Source: CAD feature listing. Evaluate the final solid. Frame: model axes, mm. A direction names the side the tool comes from. Give positions to 0.01 mm unless a question says otherwise; leave off trailing zeros. Write each loop counter-clockwise with the first axis right and the second up, starting at its lowest first coordinate (ties: lowest second). Pieces come first, ordered by that corner, then holes. Notation, with made-up numbers: (10, -7.5) -> (14, -7.5) arc R18 ccw to (14, 3.5) -> close; hole circle Ø2 at (84.25, 60). An arc over 180 degrees is marked (long way). Write item = value, one per line.
from build123d import *

# Parameters (mm, degrees)
SKETCH1_W                    = 75
SKETCH1_H                    = 139.2
SKETCH1_R                    = 1.1
SKETCH1_W_2                  = 55
SKETCH1_H_2                  = 119.2
BOSS_EXTRUDE1_DEPTH          = 0.8
BOSS_EXTRUDE1_DEPTH_BACK     = 0.8
SKETCH2_W                    = 20
SKETCH2_H                    = 10
BOSS_EXTRUDE2_DEPTH          = 1.6
SKETCH6_W                    = 125
SKETCH6_H                    = 75.4
SKETCH6_W_2                  = 105
SKETCH6_H_2                  = 55.4
BOSS_EXTRUDE4_DEPTH          = 1.6
M2_5_CLEARANCE_HOLE1_D       = 2.9
M2_5_CLEARANCE_HOLE1_DEPTH   = 11.5
FILLET1_R                    = 1.5
CUT_EXTRUDE2_DEPTH           = 10
SKETCH10_W                   = 55
SKETCH10_H                   = 10
BOSS_EXTRUDE5_DEPTH          = 1.6
SKETCH11_W                   = 19
SKETCH11_H                   = 8
SKETCH11_R                   = 1.45
BOSS_EXTRUDE6_DEPTH          = 1.6
SKETCH12_W                   = 55
SKETCH12_H                   = 8
BOSS_EXTRUDE7_DEPTH          = 1.6
FILLET3_R                    = 2
CHAMFER1_SIZE                = 5
SKETCH13_R                   = 1.5
CUT_EXTRUDE3_DEPTH           = 10
SKETCH15_R                   = 1.55
CUT_EXTRUDE4_DEPTH           = 10
CHAMFER2_SIZE                = 5
FILLET4_R                    = 2
SKETCH17_W                   = 58.67264252
SKETCH17_H                   = 24.596391624
SKETCH17_W_2                 = 62.115544984
SKETCH17_H_2                 = 8.350438831
BOSS_EXTRUDE8_DEPTH          = 1.6
SKETCH18_R                   = 0.85
CUT_EXTRUDE5_DEPTH           = 10
M2_CLEARANCE_HOLE1_D         = 2.4
M2_CLEARANCE_HOLE1_DEPTH     = 10
ESQUISSE1_R                  = 0.9
ENL_V_MAT_EXTRU_1_DEPTH      = 10
ENL_V_MAT_EXTRU_1_DEPTH_BACK = 10


with BuildPart() as part:
    # Sketch1 → Boss-Extrude1 (new body, two sides)
    with BuildSketch(Plane(origin=(0, 0, 0), x_dir=(1, 0, 0), z_dir=(0, 1, 0))) as boss_extrude1_sk:
        Rectangle(SKETCH1_W, SKETCH1_H)
        with Locations((-26.35, 64.6)):
            Circle(SKETCH1_R, mode=Mode.SUBTRACT)
        with Locations((26.35, 64.6)):
            Circle(SKETCH1_R, mode=Mode.SUBTRACT)
        with Locations((26.35, -64.6)):
            Circle(SKETCH1_R, mode=Mode.SUBTRACT)
        with Locations((-26.35, -64.6)):
            Circle(SKETCH1_R, mode=Mode.SUBTRACT)
        Rectangle(SKETCH1_W_2, SKETCH1_H_2, mode=Mode.SUBTRACT)
    extrude(amount=BOSS_EXTRUDE1_DEPTH)
    extrude(boss_extrude1_sk.sketch, amount=-BOSS_EXTRUDE1_DEPTH_BACK)

    # Sketch2 → Boss-Extrude2 (add)
    with BuildSketch(Plane(origin=(0, 0.8, 0), x_dir=(1, 0, 0), z_dir=(0, 1, 0))):
        with Locations((47.5, 49.6)):
            Rectangle(SKETCH2_W, SKETCH2_H)
        with Locations((-47.5, 49.6)):
            Rectangle(SKETCH2_W, SKETCH2_H)
        with Locations((47.5, -20.4)):
            Rectangle(SKETCH2_W, SKETCH2_H)
        with Locations((-47.5, -20.4)):
            Rectangle(SKETCH2_W, SKETCH2_H)
    extrude(amount=-BOSS_EXTRUDE2_DEPTH)

    # Sketch6 → Boss-Extrude4 (add)
    with BuildSketch(Plane(origin=(0, 0.8, 0), x_dir=(1, 0, 0), z_dir=(0, 1, 0))):
        with Locations((0, 82.3)):
            Rectangle(SKETCH6_W, SKETCH6_H)
        with Locations((0, 82.3)):
            Rectangle(SKETCH6_W_2, SKETCH6_H_2, mode=Mode.SUBTRACT)
    extrude(amount=-BOSS_EXTRUDE4_DEPTH)

    # M2.5 Clearance Hole1
    with Locations(Plane(origin=(0, 0.8, 0), x_dir=(-1, 0, 0), z_dir=(0, 1, 0))):
        with Locations((-52.5, -49.6), (-52.5, 20.4), (-42.5, -49.6), (-42.5, 20.4)):
            m2_5_clearance_hole1 = Hole(M2_5_CLEARANCE_HOLE1_D / 2, depth=M2_5_CLEARANCE_HOLE1_DEPTH)

    # Mirror1: M2.5 Clearance Hole1 across plane
    add(m2_5_clearance_hole1.mirror(Plane(origin=(0, 0, 0), x_dir=(0, 0, 1), z_dir=(1, 0, 0))), mode=Mode.SUBTRACT)

    # Fillet1
    fillet1_edges = [part.edges().sort_by_distance(p)[0] for p in [
        (37.5, 0, 25.4),
        (37.5, 0, 15.4),
        (-37.5, 0, 15.4),
        (-37.5, 0, 25.4),
        (-37.5, 0, -44.6),
        (37.5, 0, -44.6),
        (27.5, 0, -59.6),
        (-27.5, 0, -59.6),
        (27.5, 0, -54.6),
        (-27.5, 0, -54.6),
    ]]
    fillet(fillet1_edges, radius=FILLET1_R)

    # Sketch9 → Cut-Extrude2 (cut)
    with BuildSketch(Plane(origin=(0, 0.8, 0), x_dir=(1, 0, 0), z_dir=(0, 1, 0))):
        with BuildLine():
            Line((-25.25, -63.1), (-25.25, -66.1))
            ThreePointArc((-25.25, -66.1), (-26.35, -67.2), (-27.45, -66.1))
            Line((-27.45, -66.1), (-27.45, -63.1))
            ThreePointArc((-27.45, -63.1), (-26.35, -62), (-25.25, -63.1))
        make_face()
    cut_extrude2 = extrude(amount=-CUT_EXTRUDE2_DEPTH, mode=Mode.SUBTRACT)

    # Mirror2: Cut-Extrude2 across plane
    add(cut_extrude2.mirror(Plane(origin=(0, 0, 0), x_dir=(0, 0, 1), z_dir=(1, 0, 0))), mode=Mode.SUBTRACT)

    # Sketch10 → Boss-Extrude5 (add)
    with BuildSketch(Plane(origin=(0, 0.8, 0), x_dir=(1, 0, 0), z_dir=(0, 1, 0))):
        with Locations((0, -20.4)):
            Rectangle(SKETCH10_W, SKETCH10_H)
    extrude(amount=-BOSS_EXTRUDE5_DEPTH)

    # Sketch11 → Boss-Extrude6 (add)
    with BuildSketch(Plane(origin=(0, 0.8, 0), x_dir=(1, 0, 0), z_dir=(0, 1, 0))):
        with Locations((-37, 5.6)):
            Rectangle(SKETCH11_W, SKETCH11_H)
        with Locations((37, 5.6)):
            Rectangle(SKETCH11_W, SKETCH11_H)
        with Locations((42.5, 5.6)):
            Circle(SKETCH11_R, mode=Mode.SUBTRACT)
    extrude(amount=-BOSS_EXTRUDE6_DEPTH)

    # Sketch12 → Boss-Extrude7 (add)
    with BuildSketch(Plane(origin=(0, 0.8, 0), x_dir=(1, 0, 0), z_dir=(0, 1, 0))):
        with Locations((0, 5.6)):
            Rectangle(SKETCH12_W, SKETCH12_H)
    extrude(amount=-BOSS_EXTRUDE7_DEPTH)

    # Fillet3
    fillet3_edges = [part.edges().sort_by_distance(p)[0] for p in [
        (37.5, 0, -1.6),
        (-37.5, 0, -1.6),
    ]]
    fillet(fillet3_edges, radius=FILLET3_R)

    # Chamfer1
    chamfer1_edges = [part.edges().sort_by_distance(p)[0] for p in [
        (62.5, 0, -44.6),
        (62.5, 0, -120),
        (-62.5, 0, -120),
        (-62.5, 0, -44.6),
    ]]
    chamfer(chamfer1_edges, length=CHAMFER1_SIZE)

    # Sketch13 → Cut-Extrude3 (cut)
    with BuildSketch(Plane(origin=(0, 0.8, 0), x_dir=(1, 0, 0), z_dir=(0, 1, 0))):
        with Locations((-51.439339828, 108.939339828)):
            Circle(SKETCH13_R)
        with Locations((51.439339828, 108.939339828)):
            Circle(SKETCH13_R)
    extrude(amount=-CUT_EXTRUDE3_DEPTH, mode=Mode.SUBTRACT)

    # Sketch15 → Cut-Extrude4 (cut)
    with BuildSketch(Plane.XZ.offset(0.8)):
        with Locations((37, -5.6)):
            Circle(SKETCH15_R)
    cut_extrude4 = extrude(amount=-CUT_EXTRUDE4_DEPTH, mode=Mode.SUBTRACT)

    # Mirror3: Cut-Extrude4 across plane
    add(cut_extrude4.mirror(Plane(origin=(0, 0, 0), x_dir=(0, 0, 1), z_dir=(1, 0, 0))), mode=Mode.SUBTRACT)

    # Chamfer2
    chamfer2_edges = [part.edges().sort_by_distance(p)[0] for p in [
        (-27.5, 0, 59.6),
        (27.5, 0, 59.6),
        (52.5, 0, -54.6),
        (37.5, 0, -54.6),
        (-37.5, 0, -54.6),
        (-52.5, 0, -54.6),
        (27.5, 0, -44.6),
        (-27.5, 0, -44.6),
        (-27.5, 0, 15.4),
        (27.5, 0, 15.4),
        (27.5, 0, 25.4),
        (-27.5, 0, 25.4),
        (-27.5, 0, -9.6),
        (27.5, 0, -9.6),
        (27.5, 0, -1.6),
        (-27.5, 0, -1.6),
    ]]
    chamfer(chamfer2_edges, length=CHAMFER2_SIZE)

    # Fillet4
    fillet4_edges = [part.edges().sort_by_distance(p)[0] for p in [
        (-27.5, 0, 30.4),
        (-22.5, 0, 25.4),
        (-22.5, 0, -1.6),
        (-27.5, 0, 3.4),
        (-22.5, 0, 15.4),
        (-27.5, 0, 10.4),
        (-22.5, 0, -9.6),
        (-27.5, 0, -14.6),
        (-27.5, 0, -39.6),
        (-22.5, 0, -44.6),
        (37.5, 0, -59.6),
        (42.5, 0, -54.6),
        (47.5, 0, -54.6),
        (52.5, 0, -59.6),
        (22.5, 0, -44.6),
        (27.5, 0, -39.6),
        (22.5, 0, -9.6),
        (27.5, 0, -14.6),
        (22.5, 0, 15.4),
        (27.5, 0, 10.4),
        (27.5, 0, 3.4),
        (22.5, 0, -1.6),
        (27.5, 0, 30.4),
        (22.5, 0, 25.4),
        (22.5, 0, 59.6),
        (27.5, 0, 54.6),
        (-27.5, 0, 54.6),
        (-22.5, 0, 59.6),
        (-52.5, 0, -59.6),
        (-47.5, 0, -54.6),
        (-42.5, 0, -54.6),
        (-37.5, 0, -59.6),
    ]]
    fillet(fillet4_edges, radius=FILLET4_R)

    # Sketch17 → Boss-Extrude8 (add)
    with BuildSketch(Plane(origin=(0, 0.8, 0), x_dir=(1, 0, 0), z_dir=(0, 1, 0))):
        with Locations((0.384318619, -6.570339181)):
            Rectangle(SKETCH17_W, SKETCH17_H)
        with Locations((0.147528901, 56.270374441)):
            Rectangle(SKETCH17_W_2, SKETCH17_H_2)
    extrude(amount=-BOSS_EXTRUDE8_DEPTH)

    # Sketch18 → Cut-Extrude5 (cut)
    with BuildSketch(Plane(origin=(0, 0.8, 0), x_dir=(1, 0, 0), z_dir=(0, 1, 0))):
        with Locations((-37.5, 10.45)):
            Circle(SKETCH18_R)
        with Locations((37.5, 10.45)):
            Circle(SKETCH18_R)
    extrude(amount=-CUT_EXTRUDE5_DEPTH, mode=Mode.SUBTRACT)

    # M2 Clearance Hole1
    with Locations(Plane.XZ.offset(0.8)):
        with Locations((33.75, -65.6), (-33.75, -65.6)):
            Hole(M2_CLEARANCE_HOLE1_D / 2, depth=M2_CLEARANCE_HOLE1_DEPTH)

    # Esquisse1 → Enl_v. mat.-Extru.1 (cut, two sides)
    with BuildSketch(Plane.XZ.offset(0.8)) as enl_v_mat_extru_1_sk:
        with Locations((42.5, -115)):
            Circle(ESQUISSE1_R)
        with Locations((-42.5, -115)):
            Circle(ESQUISSE1_R)
    extrude(amount=ENL_V_MAT_EXTRU_1_DEPTH, mode=Mode.SUBTRACT)
    extrude(enl_v_mat_extru_1_sk.sketch, amount=-ENL_V_MAT_EXTRU_1_DEPTH_BACK, mode=Mode.SUBTRACT)


solid = part.part
(1) Section query B-B (z = -87). Return loops of the section in (x, y), plus the area to 3 significant figures.
Values follow:
outline = (-62.5, -0.8) -> (-52.5, -0.8) -> (-52.5, 0.8) -> (-62.5, 0.8) -> close; (52.5, -0.8) -> (62.5, -0.8) -> (62.5, 0.8) -> (52.5, 0.8) -> close
area = 32.0 mm2
(2) Section query D-D (y = 0.15). Give the number of separate pieces and of enclosed holes in the cut face, plus the area to 3 significant figures.
Values follow:
separate_pieces = 1
enclosed_holes = 22
area = 10,000 mm2
(3) Material intervals for line 1 (Z direction, x = -2, y = 0.65); line 2 (X direction, y = 0.4, z = 37); line 3 (X direction, y = 0.1, z = -115), sorted ascending.
Values follow:
line_1 = -120 to -110, -69.6 to -44.6, -9.6 to 25.4, 59.6 to 69.6
line_2 = -37.5 to -27.5, 27.5 to 37.5
line_3 = -62.5 to -43.4, -41.6 to 41.6, 43.4 to 62.5
(4) First-contact query: pin 1 (1.4 mm diameter, centred on x = 33.75, z = -65.6, fed in from -Y); pin 2 (0.5 mm diameter, centred on y = 0, z = -24, fed in from -X); pin 3 (0.8 mm diameter, centred on y = 0, z = 40.5, fed in from +X); pin 4 (0.8 mm diameter, centred on x = 46, y = 0, fed in from +Z). Flat tips, straight axial feed; report the tip coordinate or a pass-through.
Values follow:
pin_1 = through
pin_2 = -37.5
pin_3 = 37.5
pin_4 = 25.4
(5) Pull-direction query (Z, two-part tool) for faces 3 (the face through (-60, 0, -117.5)), 4 (the face through (-1, -0.8, -48)), 5 (the face through (25, 0, 57.1)); classes: pulls with the +Z half, pulls with the -Z half, needs draft (parallel to the pull), parting line crosses it, or undercut.
Values follow:
face_3 = pulls with the -Z half
face_4 = needs draft
face_5 = undercut
(6) Section query C-C (x = 8). Return loops of the section in (y, z).
Values follow:
outline = (-0.8, -120) -> (0.8, -120) -> (0.8, -110) -> (-0.8, -110) -> close; (-0.8, -69.6) -> (0.8, -69.6) -> (0.8, -44.6) -> (-0.8, -44.6) -> close; (-0.8, -9.6) -> (0.8, -9.6) -> (0.8, 25.4) -> (-0.8, 25.4) -> close; (-0.8, 59.6) -> (0.8, 59.6) -> (0.8, 69.6) -> (-0.8, 69.6) -> close
(7) Access query for faces 1 (the face through (60, 0, -117.5)), 2 (the face through (40, 0, -57.1)). Directions: +Z, -Z, +X, -X, +Y, -Y. A direction counts if a zero-diameter tool reaches every point of the face in a straight line with its end or side. Return the directions, or none.
Values follow:
face_1 = -Z, +X, +Y, -Y
face_2 = +Y, -Y
(8) Section query A-A (x = -29.5). Return loops of the section in (y, z).
Values follow:
outline = (-0.8, -120) -> (0.8, -120) -> (0.8, -110) -> (-0.8, -110) -> close; (-0.8, -69.6) -> (0.8, -69.6) -> (0.8, 69.6) -> (-0.8, 69.6) -> close
